```python
from build123d import *

# Parameters (mm, degrees)
CROQUIS1_W              = 40
CROQUIS1_H              = 38.3
SALIENTE_EXTRUIR1_DEPTH = 19.7
SALIENTE_EXTRUIR2_DEPTH = 2
CROQUIS3_R              = 5.9
SALIENTE_EXTRUIR3_DEPTH = 2
CROQUIS4_R              = 2.85
SALIENTE_EXTRUIR4_DEPTH = 3.5
SALIENTE_EXTRUIR5_DEPTH = 3.5


with BuildPart() as part:
    # Croquis1 → Saliente-Extruir1 (new body)
    with BuildSketch(Plane(origin=(0, 0, 0), x_dir=(0, 0, -1), z_dir=(1, 0, 0))):
        with Locations((20, 19.15)):
            Rectangle(CROQUIS1_W, CROQUIS1_H)
    extrude(amount=SALIENTE_EXTRUIR1_DEPTH)

    # Croquis2 → Saliente-Extruir2 (add)
    with BuildSketch(Plane(origin=(0, 38.3, 0), x_dir=(1, 0, 0), z_dir=(0, 1, 0))):
        with BuildLine():
            Line((0, 5.6), (19.7, 5.6))
            Line((19.7, 5.6), (19.7, 26.483687959))
            ThreePointArc((19.7, 26.483687959), (9.85, 41), (0, 26.483687959))
            Line((0, 26.483687959), (0, 5.6))
        make_face()
    extrude(amount=SALIENTE_EXTRUIR2_DEPTH)

    # Croquis3 → Saliente-Extruir3 (add)
    with BuildSketch(Plane(origin=(0, 40.3, 0), x_dir=(1, 0, 0), z_dir=(0, 1, 0))):
        with Locations(Location((9.85, 30.4, 0), (0, 0, 270))):
            Circle(CROQUIS3_R)
    extrude(amount=SALIENTE_EXTRUIR3_DEPTH)

    # Croquis4 → Saliente-Extruir4 (add)
    with BuildSketch(Plane(origin=(0, 42.3, 0), x_dir=(1, 0, 0), z_dir=(0, 1, 0))):
        with Locations(Location((9.85, 30.4, 0), (0, 0, 270))):
            Circle(CROQUIS4_R)
    extrude(amount=SALIENTE_EXTRUIR4_DEPTH)

    # Croquis5 → Saliente-Extruir5 (add)
    with BuildSketch(Plane(origin=(0, 32.4, 0), x_dir=(1, 0, 0), z_dir=(0, 1, 0))):
        with BuildLine():
            Line((0, 0), (19.7, 0))
            Line((19.7, 0), (19.7, -7))
            Line((19.7, -7), (15.65, -7))
            Line((15.65, -7), (15.65, -5.866590212))
            ThreePointArc((15.65, -5.866590212), (14.5, -1.9), (13.35, -5.866590212))
            Line((13.35, -5.866590212), (13.35, -7))
            Line((13.35, -7), (6.35, -7))
            Line((6.35, -7), (6.35, -5.866590212))
            ThreePointArc((6.35, -5.866590212), (5.2, -1.9), (4.05, -5.866590212))
            Line((4.05, -5.866590212), (4.05, -7))
            Line((4.05, -7), (0, -7))
            Line((0, -7), (0, 0))
        make_face()
        with BuildLine():
            Line((0, 40), (19.7, 40))
            Line((19.7, 40), (19.7, 47))
            Line((19.7, 47), (15.65, 47))
            Line((15.65, 47), (15.65, 45.866590212))
            ThreePointArc((15.65, 45.866590212), (14.5, 41.9), (13.35, 45.866590212))
            Line((13.35, 45.866590212), (13.35, 47))
            Line((13.35, 47), (6.35, 47))
            Line((6.35, 47), (6.35, 45.866590212))
            ThreePointArc((6.35, 45.866590212), (5.2, 41.9), (4.05, 45.866590212))
            Line((4.05, 45.866590212), (4.05, 47))
            Line((4.05, 47), (0, 47))
            Line((0, 47), (0, 40))
        make_face()
    extrude(amount=-SALIENTE_EXTRUIR5_DEPTH)


solid = part.part
```
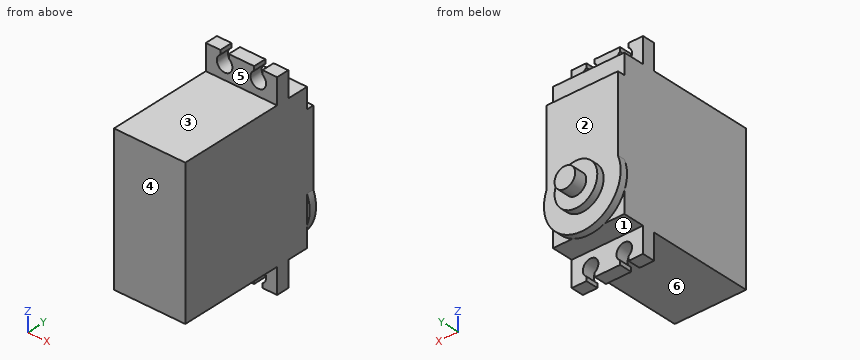
The listing builds one solid part. Answer for the finished solid, in the listing's coordinates (mm). Face numbers are marked on the shaded views. A direction names the side the tool comes from. Give positions to 0.01 mm unless a question says otherwise; leave off trailing zeros. Loops run counter-clockwise (first coordinate to the right, second up) from the corner with the lowest first, then second, coordinate; pieces in that order, holes last. Notation, with made-up numbers: M 67,-22.75 L 91,-22.75 A14 cw 91,-17.75 Z; hole C 42.5,-36 d7. An arc over 180 degrees is marked long. One line per item, written item: value.
1. Section D-D on y = 25.5 is taken. Determine the outline of the cut face in (x, z), plus the area to 3 significant figures.
Found:
outline: M 0,-40 L 19.7,-40 L 19.7,0 L 0,0 Z
area: 788 mm^2
2. For a pull along Y with two mould halves and no side action, classify the marked faces 1, 2 and 3 as pulls with the +Y half, pulls with the -Y half, needs draft (parallel to the pull), parting line crosses it, or undercut.
Found:
face 1: undercut
face 2: pulls with the +Y half
face 3: needs draft
3. Each of these flat-tipped pins is pushed along its axis until it touches: P1, Ø10, axis at x = 9.5, y = 9, coming from the -Z side; P2, Ø1.5, axis at y = 30.5, z = -21.5, coming from the +X side; P3, Ø0.9, axis at y = 30, z = -46, coming from the -X side. Where does it stop, or does it pass through?
Found:
P1: z = -40
P2: x = 19.7
P3: x = 0
4. Section C-C on z = -30.4 is taken. Determine the outline of the cut face in (x, y), plus the area to 3 significant figures.
Found:
outline: M -0.75,38.3 L 0,38.3 L 0,0 L 19.7,0 L 19.7,38.3 L 20.45,38.3 L 20.45,40.3 L 15.75,40.3 L 15.75,42.3 L 12.7,42.3 L 12.7,45.8 L 7,45.8 L 7,42.3 L 3.95,42.3 L 3.95,40.3 L -0.75,40.3 Z
area: 840 mm^2
5. For the marked faces 4, 5 and 6, determine the directions among +Z, -Z, +X, -X, +Y, -Y from which every point of the face is accessible in a straight line to the end or side of a thin tool.
Found:
face 4: +Z, -Z, +X, -X, -Y
face 5: +Z, +X, -X, -Y
face 6: -Z, +X, -X, -Y
6. Section A-A on z = -44.05 is taken. Determine the outline of the cut face in (x, y).
Found:
outline: M 0,28.9 L 3.05,28.9 L 3.05,32.4 L 0,32.4 Z; M 7.35,28.9 L 12.35,28.9 L 12.35,32.4 L 7.35,32.4 Z; M 16.65,28.9 L 19.7,28.9 L 19.7,32.4 L 16.65,32.4 Z
7. Find the intervals of material crossed by probe 1 along X at (y, z) = (31, 4); probe 2 along Z at (x, y) = (14.5, 31.15); probe 3 along Z at (x, y) = (3.25, 15), in increasing order.
Found:
probe 1: 0 to 3.05, 7.35 to 12.35, 16.65 to 19.7
probe 2: -41.9 to 1.9
probe 3: -40 to 0
8. Section B-B on x = 9.85 is taken. Determine the outline of the cut face in (y, z), plus the area to 3 significant figures.
Found:
outline: M 0,-40 L 28.9,-40 L 28.9,-47 L 32.4,-47 L 32.4,-40 L 38.3,-40 L 38.3,-41 L 40.3,-41 L 40.3,-36.3 L 42.3,-36.3 L 42.3,-33.25 L 45.8,-33.25 L 45.8,-27.55 L 42.3,-27.55 L 42.3,-24.5 L 40.3,-24.5 L 40.3,-5.6 L 38.3,-5.6 L 38.3,0 L 32.4,0 L 32.4,7 L 28.9,7 L 28.9,0 L 0,0 Z
area: 1,700 mm^2
